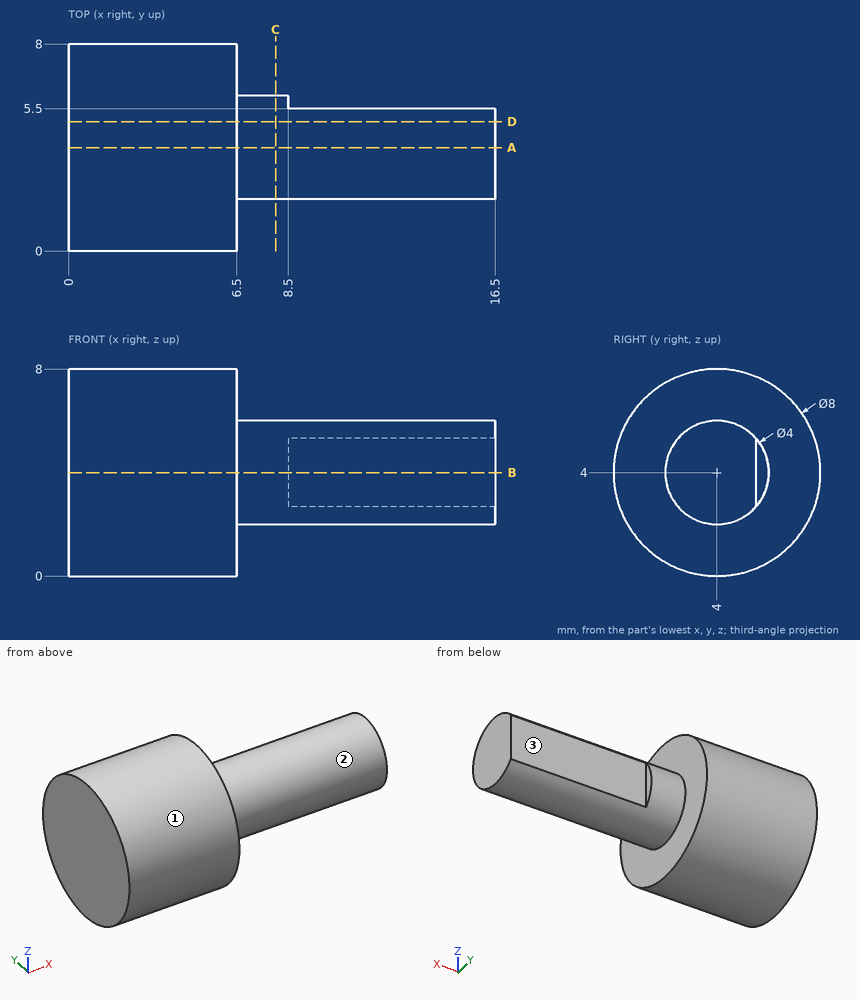
Study the drawing (mm; zero at the part's minimum x, y, z) and answer. A direction names the side the tool comes from. Round coordinates to 2 decimals unless told otherwise and drop trailing zeros. Loops run counter-clockwise (first coordinate to the right, second up) from the corner with the lowest first, then second, coordinate; pieces in that order, holes last. Notation, with made-up numbers: (41, 19.5) -> (82, 19.5) arc R6 cw to (82, 29.5) -> close; hole circle Ø4 at (75, -12.5). An arc over 180 degrees is marked (long way). Use one line per item in the form item = value.
1. A tool of negligible diameter and unlimited length cuts with its end or side. For the marked faces 1, 2 and 3, from which of +Z, -Z, +X, -X, +Y, -Y can it reach the whole face along a straight path? Write none if from no direction.
Answer key:
face_1 = +X, -X
face_2 = +X
face_3 = +Z, -Z, +X, +Y
2. The part is cut by section D-D on y = 5. Determine the outline of the cut face in (x, z), and give its area (3 significant figures).
Answer key:
outline = (0, 0.13) -> (6.5, 0.13) -> (6.5, 2.27) -> (16.5, 2.27) -> (16.5, 5.73) -> (6.5, 5.73) -> (6.5, 7.87) -> (0, 7.87) -> close
area = 85.0 mm²
3. Find the intervals of material crossed by probe 1 along X at (y, z) = (6.25, 6.25); probe 2 along Y at (x, z) = (11, 5.5); probe 3 along Y at (x, z) = (13.75, 3.75), in increasing order. Write a range as [from, to].
Answer key:
probe_1 = [0, 6.5]
probe_2 = [2.68, 5.32]
probe_3 = [2.02, 5.5]
4. The part is cut by section B-B on z = 4. Determine the outline of the cut face in (x, y).
Answer key:
outline = (0, 0) -> (6.5, 0) -> (6.5, 2) -> (16.5, 2) -> (16.5, 5.5) -> (8.5, 5.5) -> (8.5, 6) -> (6.5, 6) -> (6.5, 8) -> (0, 8) -> close
5. The part is cut by section C-C on x = 8. Determine the outline of the cut face in (y, z), and give its area (3 significant figures).
Answer key:
outline = circle Ø4 at (4, 4)
area = 12.6 mm²
6. The part is cut by section A-A on y = 4. Determine the outline of the cut face in (x, z), and give its area (3 significant figures).
Answer key:
outline = (0, 0) -> (6.5, 0) -> (6.5, 2) -> (16.5, 2) -> (16.5, 6) -> (6.5, 6) -> (6.5, 8) -> (0, 8) -> close
area = 92.0 mm²
7. Flat-ended cylindrical pins translate along their axes: pin 1 Ø1.5 at (y, z) = (7, 1.5) entering from +X; pin 2 Ø2 at (x, z) = (8.5, 4) entering from -Y; pin 3 Ø2 at (x, z) = (11.5, 4.5) entering from +Y. Find the tip coordinate at first contact, or state that the pin passes through.
Answer key:
pin_1 = 6.5
pin_2 = 2
pin_3 = 5.5
